Verification items for the finished model (mm, model axes). Coordinates: 2 decimals unless noted, no trailing zeros. Write each loop counter-clockwise with the first axis right and the second up, starting at its lowest first coordinate (ties: lowest second). Pieces come first, ordered by that corner, then holes.
```python
from build123d import *

# Parameters (mm, degrees)
F0_R     = 12.7
F1_DEPTH = 25.4
F2_R     = 12.7
F3_DEPTH = 25.4
F4_R     = 5.08


with BuildPart() as f1:
    # F0 (on Front) → F1 (new body)
    with BuildSketch(Plane.XZ):
        with BuildLine():
            Line((75.0824, -18.542002), (-12.279727, 40.592327))
            ThreePointArc((-12.279727, 40.592327), (-38.423859, 41.994598), (-51.9176, 19.557998))
            Line((-51.9176, 19.557998), (-51.9176, -31.242002))
            Line((-51.9176, -31.242002), (75.0824, -31.242002))
            Line((75.0824, -31.242002), (75.0824, -18.542002))
        make_face()
        with Locations((-26.5176, 19.557998)):
            Circle(F0_R, mode=Mode.SUBTRACT)
    extrude(amount=F1_DEPTH)

    # F2 (on face) → F3 (join)
    with BuildSketch(Plane.XZ.offset(25.4)):
        with BuildLine():
            Line((75.0824, -31.242002), (75.0824, -18.542002))
            Line((75.0824, -18.542002), (-1.233405, -18.542002))
            Line((-1.233405, -18.542002), (-1.233405, 17.13529))
            ThreePointArc((-1.233405, 17.13529), (-3.538118, 30.379431), (-12.279727, 40.592327))
            ThreePointArc((-12.279727, 40.592327), (-38.423859, 41.994598), (-51.9176, 19.557998))
            Line((-51.9176, 19.557998), (-51.9176, -18.542002))
            Line((-51.9176, -18.542002), (-51.9176, -31.242002))
            Line((-51.9176, -31.242002), (75.0824, -31.242002))
        make_face()
        with Locations((-26.5176, 19.557998)):
            Circle(F2_R, mode=Mode.SUBTRACT)
    extrude(amount=F3_DEPTH)

    # F4
    f4_edges = [f1.edges().sort_by_distance(p)[0] for p in [
        (75.0824, -50.8, -24.892002),
    ]]
    fillet(f4_edges, radius=F4_R)


solid = f1.part
```
1. Sectioned sample at C-C, the plane x = -18. Record the boundary of the cut face in (y, z).
2. Draft check along Z on faces 1 (the cylindrical face through (-36.596, -25.044, 11.83)), 2 (the flat face through (32.013, -12.522, 10.611)), 3 (the flat face through (-1.233, -38, -1)), 4 (the flat face through (75.082, -23, -25)). Enter one of: pulls with the +Z half, pulls with the -Z half, needs draft (parallel to the pull), parting line crosses it, or undercut.
3. Sectioned sample at B-B, the plane z = 8.5. Record the boundary of the cut face in (x, y).
4. Gauge pin test, flat ends, axial feed: P1, Ø1, axis at x = 56, z = -21.5, coming from the +Y side; P2, Ø1, axis at x = 62, z = -14, coming from the -Y side; P3, Ø12, axis at x = 37.5, z = 20.5, coming from the +Y side; P4, Ø20.5, axis at x = 46, y = -40.5, coming from the +Z side. Record the tip position at first contact, or that the pin passes through.
5. Sectioned sample at D-D, the plane x = 12. Record the boundary of the cut face in (y, z), and give its area (3 significant figures).
6. Material ranges on L1, parallel to X at y = -27, z = 19; L2, parallel to Z at x = -29, y = -36; L3, parallel to X at y = -29, z = 21.5, recorded low to high.
7. Sectioned sample at A-A, the plane y = -37. Record the boundary of the cut face in (x, z).
Outcome:
1. outline: (-50.8, -31.24) - (0, -31.24) - (0, 10.14) - (-50.8, 10.14) - close; (-50.8, 28.98) - (0, 28.98) - (0, 43.49) - (-50.8, 43.49) - close
2. face 1: undercut
2. face 2: pulls with the +Z half
2. face 3: undercut
2. face 4: needs draft
3. outline: (-51.92, -50.8) - (-32.76, -50.8) - (-32.76, 0) - (-51.92, 0) - close; (-20.27, -50.8) - (-1.23, -50.8) - (-1.23, -25.4) - (35.13, -25.4) - (35.13, 0) - (-20.27, 0) - close
4. P1: stops at y = 0
4. P2: stops at y = -25.4
4. P3: passes through
4. P4: stops at z = -18.54
5. outline: (-50.8, -31.24) - (0, -31.24) - (0, 24.16) - (-25.4, 24.16) - (-25.4, -18.54) - (-50.8, -18.54) - close
5. area: 1,730 mm2
6. L1: x = -51.92 to -39.21, -13.83 to -1.12
6. L2: z = -31.24 to 7.1, 32.01 to 44.84
6. L3: x = -51.84 to -39.07, -13.97 to -1.19
7. outline: (-51.92, -31.24) - (75.08, -31.24) - (75.08, -18.54) - (-1.23, -18.54) - (-1.23, 17.14) arc R25.4 ccw to (-12.28, 40.59) arc R25.4 ccw to (-51.92, 19.56) - close; hole circle Ø25.4 at (-26.52, 19.56)
